Geometry check sheet. Reference: the model listing, model coordinates, mm. Face numbers are marked on the shaded views. Give positions to 0.01 mm unless a question says otherwise; leave off trailing zeros. Write each loop counter-clockwise with the first axis right and the second up, starting at its lowest first coordinate (ties: lowest second). Pieces come first, ordered by that corner, then holes.
(1) Depth check by flat-ended pin: P1, Ø3, axis at x = -12.5, z = 6.5, coming from the +Y side; P2, Ø4, axis at y = 2, z = 0.5, coming from the -X side; P3, Ø17.5, axis at x = -43.3, y = 25, coming from the +Z side; P4, Ø1, axis at y = -40, z = 3, coming from the +X side. Enter the tip coordinate at first touch or a pass-through.
(2) Thickness scan on line 1 along Y through (x, z) = (-1.5, 0.5); line 2 along X through (y, z) = (29, 4.25); line 3 along X through (y, z) = (4.5, 4). Record the ranges inside material, lowest first.
(3) Cross-section at B-B (x = -40.5). Record the boundary of the cut face in (y, z).
(4) Cross-section at A-A (z = 5.75). Record the boundary of the cut face in (x, y) (3 decimals).
(5) Mould release check, pull along Y, two halves, no side actions. Record for the marked faces 1, 2 and 3: +Y half, -Y half, draft (parallel to the pull), parting line (faces both ways), or undercut.
(6) Cross-section at C-C (y = -45.5). Record the boundary of the cut face in (x, z), and give its area (3 significant figures).
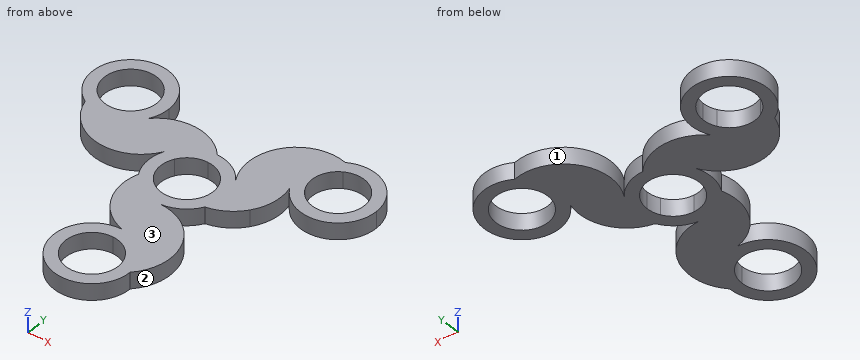
```python
from build123d import *

# Parameters (mm, degrees)
F1_DEPTH = 7


# Not quite as in the source:
# - a feature names something its author has since deleted; it is built from what else it names


with BuildPart() as f1:
    # F0 (on Top) → F1 (new body)
    with BuildSketch(Plane.XY):
        with BuildLine():
            Line((16, 0), (11, 0))
            ThreePointArc((11, 0), (10.6251840892, -2.8470094961), (9.5262794416, -5.5))
            Line((9.5262794416, -5.5), (13.8564064606, -8))
            ThreePointArc((13.8564064606, -8), (15.4548132206, -4.1411047216), (16, 0))
        make_face()
        with BuildLine():
            ThreePointArc((9.5262794416, 5.5), (10.6251840892, 2.8470094961), (11, 0))
            Line((11, 0), (16, 0))
            ThreePointArc((16, 0), (15.4548132206, 4.1411047216), (13.8564064606, 8))
            Line((13.8564064606, 8), (9.5262794416, 5.5))
        make_face()
        with BuildLine():
            ThreePointArc((0, 11), (5.5, 9.5262794416), (9.5262794416, 5.5))
            Line((9.5262794416, 5.5), (13.8564064606, 8))
            ThreePointArc((13.8564064606, 8), (13.409185793, 8.6628012124), (12.9888150126, 9.3429483874))
            ThreePointArc((12.9888150126, 9.3429483874), (7.2976991512, 14.2388056767), (0, 16))
            Line((0, 16), (0, 11))
        make_face()
        with BuildLine():
            Line((13.8564064606, -8), (9.5262794416, -5.5))
            ThreePointArc((9.5262794416, -5.5), (5.5, -9.5262794416), (0, -11))
            Line((0, -11), (0, -16))
            ThreePointArc((0, -16), (0.7976130214, -15.944096147), (1.5968231434, -15.9201179596))
            ThreePointArc((1.5968231434, -15.9201179596), (8.68231786, -13.4393956924), (13.8564064606, -8))
        make_face()
        with BuildLine():
            Line((26.4227403385, 0), (16, 0))
            ThreePointArc((16, 0), (15.4548132206, -4.1411047216), (13.8564064606, -8))
            ThreePointArc((13.8564064606, -8), (20.912199664, -5.2136349503), (26.4227403385, 0))
        make_face()
        with BuildLine():
            ThreePointArc((13.8564064606, 8), (15.4548132206, 4.1411047216), (16, 0))
            Line((16, 0), (26.4227403385, 0))
            ThreePointArc((26.4227403385, 0), (29.8628617611, 8.1570672633), (29.4448637287, 17))
            Line((29.4448637287, 17), (13.8564064606, 8))
        make_face()
        with BuildLine():
            ThreePointArc((-9.5262794416, 5.5), (-5.5, 9.5262794416), (0, 11))
            Line((0, 11), (0, 16))
            ThreePointArc((0, 16), (-8, 13.8564064606), (-13.8564064606, 8))
            Line((-13.8564064606, 8), (-9.5262794416, 5.5))
        make_face()
        with BuildLine():
            ThreePointArc((12.9888150126, 9.3429483874), (13.409185793, 8.6628012124), (13.8564064606, 8))
            ThreePointArc((13.8564064606, 8), (13.4393956924, 8.68231786), (12.9888150126, 9.3429483874))
        make_face()
        with BuildLine():
            ThreePointArc((12.9888150126, 9.3429483874), (13.4393956924, 8.68231786), (13.8564064606, 8))
            Line((13.8564064606, 8), (29.4448637287, 17))
            ThreePointArc((29.4448637287, 17), (27.8464569686, 29.1411047216), (35.3012701892, 38.8564064606))
            ThreePointArc((35.3012701892, 38.8564064606), (14.2545680685, 31.576970296), (12.9888150126, 9.3429483874))
        make_face()
        with BuildLine():
            Line((0, -16), (0, -11))
            ThreePointArc((0, -11), (-5.5, -9.5262794416), (-9.5262794416, -5.5))
            Line((-9.5262794416, -5.5), (-13.8564064606, -8))
            ThreePointArc((-13.8564064606, -8), (-8, -13.8564064606), (0, -16))
        make_face()
        with BuildLine():
            ThreePointArc((-9.5262794416, -5.5), (-11, 0), (-9.5262794416, 5.5))
            Line((-9.5262794416, 5.5), (-13.8564064606, 8))
            ThreePointArc((-13.8564064606, 8), (-14.2067988144, 7.2812949346), (-14.585638156, 6.5771695722))
            ThreePointArc((-14.585638156, 6.5771695722), (-15.9800170112, -0.7994099843), (-13.8564064606, -8))
            Line((-13.8564064606, -8), (-9.5262794416, -5.5))
        make_face()
        with BuildLine():
            ThreePointArc((-13.8564064606, 8), (-8, 13.8564064606), (0, 16))
            ThreePointArc((0, 16), (-14.5027493597, 22.9685214121), (-29.4448637287, 17))
            Line((-29.4448637287, 17), (-13.8564064606, 8))
        make_face()
        with BuildLine():
            ThreePointArc((35.3012701892, 38.8564064606), (27.8464569686, 29.1411047216), (29.4448637287, 17))
            Line((29.4448637287, 17), (33.7749907476, 19.5))
            ThreePointArc((33.7749907476, 19.5), (32.6760861, 27.8470094961), (37.8012701892, 34.5262794416))
            Line((37.8012701892, 34.5262794416), (35.3012701892, 38.8564064606))
        make_face()
        with BuildLine():
            Line((33.7749907476, 19.5), (29.4448637287, 17))
            ThreePointArc((29.4448637287, 17), (47.4423749109, 9.5451867794), (59.3012701892, 25))
            ThreePointArc((59.3012701892, 25), (51.3012701892, 38.8564064606), (35.3012701892, 38.8564064606))
            Line((35.3012701892, 38.8564064606), (37.8012701892, 34.5262794416))
            ThreePointArc((37.8012701892, 34.5262794416), (48.8012701892, 34.5262794416), (54.3012701892, 25))
            ThreePointArc((54.3012701892, 25), (46.1482796853, 14.3748159108), (33.7749907476, 19.5))
        make_face()
        with BuildLine():
            Line((0, -34), (0, -16))
            ThreePointArc((0, -16), (-8, -13.8564064606), (-13.8564064606, -8))
            ThreePointArc((-13.8564064606, -8), (-12.6399483504, -24.0440100763), (0, -34))
        make_face()
        with BuildLine():
            ThreePointArc((1.5968231434, -15.9201179596), (0.7976130214, -15.944096147), (0, -16))
            ThreePointArc((0, -16), (0.7994099843, -15.9800170112), (1.5968231434, -15.9201179596))
        make_face()
        with BuildLine():
            ThreePointArc((1.5968231434, -15.9201179596), (0.7994099843, -15.9800170112), (0, -16))
            Line((0, -16), (0, -34))
            ThreePointArc((0, -34), (11.313708499, -38.686291501), (16, -50))
            ThreePointArc((16, -50), (20.2191744167, -28.1333032153), (1.5968231434, -15.9201179596))
        make_face()
        with BuildLine():
            ThreePointArc((-14.585638156, 6.5771695722), (-14.2067988144, 7.2812949346), (-13.8564064606, 8))
            ThreePointArc((-13.8564064606, 8), (-14.2388056767, 7.2976991512), (-14.585638156, 6.5771695722))
        make_face()
        with BuildLine():
            ThreePointArc((-14.585638156, 6.5771695722), (-14.2388056767, 7.2976991512), (-13.8564064606, 8))
            Line((-13.8564064606, 8), (-29.4448637287, 17))
            ThreePointArc((-29.4448637287, 17), (-39.1601654676, 9.5451867794), (-51.3012701892, 11.1435935394))
            ThreePointArc((-51.3012701892, 11.1435935394), (-34.4737424851, -3.4436670807), (-14.585638156, 6.5771695722))
        make_face()
        with BuildLine():
            ThreePointArc((-51.3012701892, 11.1435935394), (-39.1601654676, 9.5451867794), (-29.4448637287, 17))
            Line((-29.4448637287, 17), (-33.7749907476, 19.5))
            ThreePointArc((-33.7749907476, 19.5), (-40.4542606931, 14.3748159108), (-48.8012701892, 15.4737205584))
            Line((-48.8012701892, 15.4737205584), (-51.3012701892, 11.1435935394))
        make_face()
        with BuildLine():
            Line((-33.7749907476, 19.5), (-29.4448637287, 17))
            ThreePointArc((-29.4448637287, 17), (-27.8464569686, 20.8588952784), (-27.3012701892, 25))
            ThreePointArc((-27.3012701892, 25), (-51.3012701892, 38.8564064606), (-51.3012701892, 11.1435935394))
            Line((-51.3012701892, 11.1435935394), (-48.8012701892, 15.4737205584))
            ThreePointArc((-48.8012701892, 15.4737205584), (-48.8012701892, 34.5262794416), (-32.3012701892, 25))
            ThreePointArc((-32.3012701892, 25), (-32.6760861, 22.1529905039), (-33.7749907476, 19.5))
        make_face()
        with BuildLine():
            ThreePointArc((16, -50), (11.313708499, -38.686291501), (0, -34))
            Line((0, -34), (0, -39))
            ThreePointArc((0, -39), (7.7781745931, -42.2218254069), (11, -50))
            Line((11, -50), (16, -50))
        make_face()
        with BuildLine():
            Line((0, -39), (0, -34))
            ThreePointArc((0, -34), (-11.313708499, -61.313708499), (16, -50))
            Line((16, -50), (11, -50))
            ThreePointArc((11, -50), (-7.7781745931, -57.7781745931), (0, -39))
        make_face()
    extrude(amount=F1_DEPTH)


solid = f1.part
```
Reply:
1. P1: stops at y = 22.95
1. P2: stops at x = -47.69
1. P3: passes through
1. P4: stops at x = 21.47
2. line 1: y = -65.93 to -60.9, -39.1 to -34.07, -33.55 to -10.9, 10.9 to 17.57
2. line 2: x = -58.79 to -53.55, -33.05 to -27.81, 12.6 to 33.05, 53.55 to 58.79
2. line 3: x = -48.08 to -15.93, -15.35 to -10.04, 10.04 to 28.85
3. outline: (-1.7, 0) - (14.36, 0) - (14.36, 7) - (-1.7, 7) - close; (35.64, 0) - (40.75, 0) - (40.75, 7) - (35.64, 7) - close
4. outline: (-51.301, 11.144) arc R20 ccw to (-14.586, 6.577) arc R16 ccw to (-13.856, -8) arc R20 ccw to (0, -34) arc R16 ccw (long way) to (16, -50) arc R20 ccw to (1.597, -15.92) arc R16 ccw to (13.856, -8) arc R20 ccw to (29.445, 17) arc R16 ccw (long way) to (35.301, 38.856) arc R20 ccw to (12.989, 9.343) arc R16 ccw to (0, 16) arc R20 ccw to (-29.445, 17) arc R16 ccw (long way) to start; hole circle Ø22 at (-43.301, 25); hole circle Ø22 at (0, -50); hole circle Ø22 at (0, 0); hole circle Ø22 at (43.301, 25)
5. face 1: undercut
5. face 2: undercut
5. face 3: draft
6. outline: (-15.35, 0) - (-10.04, 0) - (-10.04, 7) - (-15.35, 7) - close; (10.04, 0) - (19.35, 0) - (19.35, 7) - (10.04, 7) - close
6. area: 102 mm2
